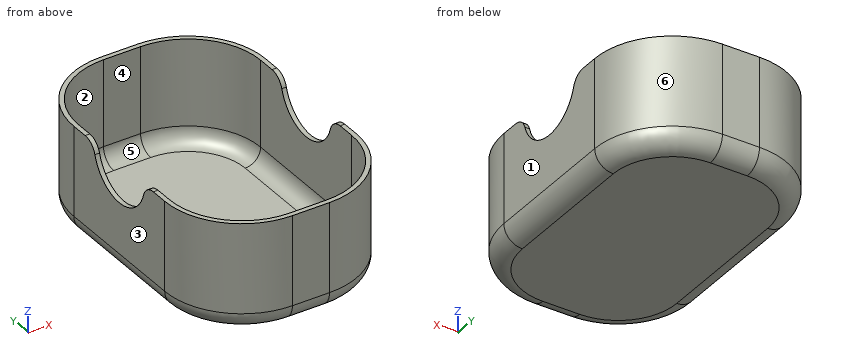
```python
from build123d import *

# Parameters (mm, degrees)
F0_W     = 62
F0_H     = 95
F1_DEPTH = 35
F2_R     = 25
F4_DEPTH = 33
F6_DEPTH = 62.001
F7_R     = 5
F8_R     = 5
F9_R     = 6


with BuildPart() as f1:
    # F0 (on Top) → F1 (new body)
    with BuildSketch(Plane.XY):
        Rectangle(F0_W, F0_H)
    extrude(amount=F1_DEPTH)

    # F2
    f2_edges = [f1.edges().sort_by_distance(p)[0] for p in [
        (31, 47.5, 17.5),
        (-31, 47.5, 17.5),
        (31, -47.5, 17.5),
        (-31, -47.5, 17.5),
    ]]
    fillet(f2_edges, radius=F2_R)

    # F3 (on face) → F4 (cut)
    with BuildSketch(Plane.XY.offset(35)):
        with BuildLine():
            Line((29.5, -22.5), (29.5, 22.5))
            ThreePointArc((29.5, 22.5), (22.6170093579, 39.1170093579), (6, 46))
            Line((6, 46), (-6, 46))
            ThreePointArc((-6, 46), (-22.6170093579, 39.1170093579), (-29.5, 22.5))
            Line((-29.5, 22.5), (-29.5, -22.5))
            ThreePointArc((-29.5, -22.5), (-22.6170093579, -39.1170093579), (-6, -46))
            Line((-6, -46), (6, -46))
            ThreePointArc((6, -46), (22.6170093579, -39.1170093579), (29.5, -22.5))
        make_face()
    extrude(amount=-F4_DEPTH, mode=Mode.SUBTRACT)

    # F5 (on face) → F6 (cut, through all)
    with BuildSketch(Plane.YZ.offset(31)):
        with BuildLine():
            ThreePointArc((-12.5715859231, 35), (0, 22.4284140769), (12.5715859231, 35))
            Line((12.5715859231, 35), (-12.5715859231, 35))
        make_face()
    extrude(amount=-F6_DEPTH, mode=Mode.SUBTRACT)

    # F7
    f7_edges = [f1.edges().sort_by_distance(p)[0] for p in [
        (30.25, 12.571586, 35),
        (-30.25, 12.571586, 35),
        (30.25, -12.571586, 35),
        (-30.25, -12.571586, 35),
    ]]
    fillet(f7_edges, radius=F7_R)

    # F8
    f8_edges = [f1.edges().sort_by_distance(p)[0] for p in [
        (-22.617009, 39.117009, 2),
    ]]
    fillet(f8_edges, radius=F8_R)

    # F9
    f9_edges = [f1.edges().sort_by_distance(p)[0] for p in [
        (31, 0, 0),
    ]]
    fillet(f9_edges, radius=F9_R)


solid = f1.part
```
CAD build for the part. Positions are in the model's coordinates, mm. Face numbers are marked on the shaded views. A direction names the side the tool comes from. Coordinates: 2 decimals unless noted, no trailing zeros. Write each loop counter-clockwise with the first axis right and the second up, starting at its lowest first coordinate (ties: lowest second). Pieces come first, ordered by that corner, then holes.
(1) Flat gauge pins, fed straight in: pin 1 (4 mm diameter, centred on x = -23, y = 35, fed in from +Z); pin 2 (6 mm diameter, centred on y = 38, z = 21.5, fed in from -X); pin 3 (1.5 mm diameter, centred on x = 23.5, z = 11.5, fed in from -Y). Where does each tip first touch, or does it go through?
(2) Cut at B-B, the plane z = 27. List the corners of the cut face in (x, y), and give its area (3 significant figures).
(3) Cut at D-D, the plane y = 18.5. List the corners of the cut face in (x, z), and give its area (3 significant figures).
(4) Drill centre lines: probe 1 along Y at (x, z) = (5, 20); probe 2 along X at (y, z) = (-4.5, 9.5); probe 3 along Z at (x, y) = (-5.5, -19.5). Where is each one in solid material? Low to high.
(5) 3-axis set-ups, long thin cutter, end or side, ignore diameter. For the marked faces 1 and 2: which of +Z, -Z, +X, -X, +Y, -Y reach the whole face in a straight line?
(6) Cut at A-A, the plane z = 15.5. List the corners of the cut face in (x, y).
(7) Cut at C-C, the plane x = 4.5. List the corners of the cut face in (y, z).
(8) Two-plate mould, pull along X, no slides. Class the marked faces 3, 4, 5 and 6: +X half, -X half, draft (parallel to the pull), parting line (faces both ways), or undercut.
Geometry says:
1. pin 1: stops at z = 5.04
1. pin 2: stops at x = -27.65
1. pin 3: stops at y = -41.06
2. outline: (-31, -22.5) arc R25 ccw to (-6, -47.5) - (6, -47.5) arc R25 ccw to (31, -22.5) - (31, -9.7) - (29.5, -9.7) - (29.5, -22.5) arc R23.5 cw to (6, -46) - (-6, -46) arc R23.5 cw to (-29.5, -22.5) - (-29.5, -9.7) - (-31, -9.7) - close; (-31, 9.7) - (-29.5, 9.7) - (-29.5, 22.5) arc R23.5 cw to (-6, 46) - (6, 46) arc R23.5 cw to (29.5, 22.5) - (29.5, 9.7) - (31, 9.7) - (31, 22.5) arc R25 ccw to (6, 47.5) - (-6, 47.5) arc R25 ccw to (-31, 22.5) - close
2. area: 341 mm2
3. outline: (-31, 6) arc R6 ccw to (-25, 0) - (25, 0) arc R6 ccw to (31, 6) - (31, 35) - (29.5, 35) - (29.5, 7) arc R5 cw to (24.5, 2) - (-24.5, 2) arc R5 cw to (-29.5, 7) - (-29.5, 35) - (-31, 35) - close
3. area: 218 mm2
4. probe 1: y = -47.5 to -46, 46 to 47.5
4. probe 2: x = -31 to -29.5, 29.5 to 31
4. probe 3: z = 0 to 2
5. face 1: +Z, -Z, +X, +Y, -Y
5. face 2: +Z
6. outline: (-31, -22.5) arc R25 ccw to (-6, -47.5) - (6, -47.5) arc R25 ccw to (31, -22.5) - (31, 22.5) arc R25 ccw to (6, 47.5) - (-6, 47.5) arc R25 ccw to (-31, 22.5) - close; hole (-29.5, -22.5) arc R23.5 ccw to (-6, -46) - (6, -46) arc R23.5 ccw to (29.5, -22.5) - (29.5, 22.5) arc R23.5 ccw to (6, 46) - (-6, 46) arc R23.5 ccw to (-29.5, 22.5) - close
7. outline: (-47.5, 6) arc R6 ccw to (-41.5, 0) - (41.5, 0) arc R6 ccw to (47.5, 6) - (47.5, 35) - (46, 35) - (46, 7) arc R5 cw to (41, 2) - (-41, 2) arc R5 cw to (-46, 7) - (-46, 35) - (-47.5, 35) - close
8. face 3: -X half
8. face 4: undercut
8. face 5: undercut
8. face 6: +X half
